Could you check a few things on this model? Use its own coordinates, in mm. A direction names the side the tool comes from. Give positions to 0.01 mm unless a question says otherwise; leave off trailing zeros. Order: outer loops, then holes, each group sorted by start corner. A loop starts at its lowest first (then second) coordinate and runs counter-clockwise, first axis right, second up.
Solid Edge part; units mm, degrees
sketch "Sketch1" plane through (0, 0, 0) normal (1, 0, 0) x (0, 1, 0)
  line L0 (0, 1.95) -> (15, 1.95)
  line L1 (15, 1.95) -> (15, 7.5)
  line L2 (15, 7.5) -> (10.5, 7.5)
  line L3 (10.5, 7.5) -> (10.5, 12.5)
  line L4 (10.5, 12.5) -> (0, 12.5)
  line L5 (0, 12.5) -> (0, 1.95)
  dimension "D1" = 10.5
  dimension "D2" = 15
revolve "RevolvedProtrusion1" add sketch "Sketch1" angle 360 about axis through (0, -60, 0) along (0, 1, 0)
chamfer "Chamfer_1" distance 0.5 angle 60 1 edges at (0, 15, 7.5) measured on face at (-4.85, 15, 5.15)
sketch "Sketch2" plane through (0, 0, 0) normal (0, -1, 0) x (1, 0, 0)
  line L0 (-7.5, 2.5) -> (7.5, 2.5)
  line L1 (7.5, 2.5) -> (10, 35)
  line L2 (10, 95) -> (10, 35)
  line L3 (-10, 95) -> (10, 95)
  line L4 (-10, 35) -> (-10, 95)
  line L5 (-10, 35) -> (-7.5, 2.5)
  dimension "D1" = 10
  dimension "D2" = 7.5
extrude "ExtrudedProtrusion_1" add sketch "Sketch2" against normal blind 9
chamfer "Chamfer_2" distance 0.5 angle 60 1 edges at (0, 0, 1.95) measured on face at (-8.0833, 0, 4.3417)
sketch "Sketch3" plane through (0, 9, 43.7496) normal (0, 1, 0) x (0, 0, -1)
  line L0 (-38.7504, 22.5) -> (-38.7504, -22.5)
  line L1 (-38.7504, -22.5) -> (6.2496, -22.5)
  line L2 (6.2496, -22.5) -> (6.2496, 22.5)
  line L3 (6.2496, 22.5) -> (-38.7504, 22.5)
  dimension "D1" = 38.7504
extrude "ExtrudedProtrusion_2" add sketch "Sketch3" against normal blind 9
sketch "Sketch4" plane through (0, 0, 36.25) normal (0, -1, 0) x (0, 0, 1)
  line L0 (1.25, -22.5) -> (46.25, -22.5)
  line L1 (46.25, -22.5) -> (46.25, 22.5)
  line L2 (46.25, 22.5) -> (1.25, 22.5)
  line L3 (1.25, 22.5) -> (1.25, -22.5)
extrude "ExtrudedCutout_1" cut sketch "Sketch4" against normal blind 3
hole "Hole_1" at (0, 3, 60) direction (0, 1, 0) diameter 8 end up to next
hole "Hole_2" at (15.5, 9, 75.5) direction (0, -1, 0) diameter 3.6 end up to next counterbore diameter 6.5 counterbore depth 4.5
hole "Hole1" at (-15.5, 9, 75.5) direction (0, -1, 0) diameter 3.6 end up to next counterbore diameter 6.5 counterbore depth 4.5
hole "Hole2" at (-15.5, 9, 44.5) direction (0, -1, 0) diameter 3.6 end up to next counterbore diameter 6.5 counterbore depth 4.5
hole "Hole3" at (15.5, 9, 44.5) direction (0, -1, 0) diameter 3.6 end up to next counterbore diameter 6.5 counterbore depth 4.5
sketch "Sketch5" plane through (0, 4.5, 95) normal (0, 0, 1) x (0, 1, 0)
  line L0 (-4.5, 10) -> (0, 10)
  line L1 (0, 10) -> (0, -10)
  line L2 (0, -10) -> (-4.5, -10)
  line L3 (-4.5, -10) -> (-4.5, 10)
extrude "ExtrudedCutout_2" cut sketch "Sketch5" against normal blind 12.5
hole "Hole_6" at (5, 9, 88.75) direction (0, -1, 0) diameter 5 end up to next
hole "Hole4" at (-5, 9, 88.75) direction (0, -1, 0) diameter 5 end up to next
chamfer "Chamfer_3" distance 3 angle 45 4 edges at (22.5, 6, 37.5) (22.5, 6, 82.5) (-22.5, 6, 82.5) (-22.5, 6, 37.5)
chamfer "Chamfer_4" distance 2 angle 45 1 edges at (0, 0, 37.5)
hole "Hole_8" at (0, 3, 60) direction (0, 1, 0) diameter 22 depth 50.8
chamfer "Chamfer_5" distance 0.5 angle 45 1 edges at (0, 3, 71)
properties material "Polyethylene, low density"
Item 1: We'd pull the mould along X, two halves only. Please class faces 1 (the flat face through (10, 7, 89)), 2 (the flat face through (-1.5, 15, 1.5)), 3 (the cylindrical face through (16.717, 3.761, 74.173)): +X half, -X half, draft (parallel to the pull), parting line (faces both ways), or undercut.
Findings:
face 1: +X half
face 2: draft
face 3: undercut
Item 2: Imagine slicing it at B-B on x = 0. Give the number of separate pieces and of enclosed holes in the cut face, then the cut area to 3 significant figures.
Findings:
separate pieces: 3
enclosed holes: 0
area: 688 mm2
Item 3: Please list where these lines run through material, in increasing order: line 1 along Z through (x, y) = (15.5, 6.5); line 2 along X through (y, z) = (3.75, 44.5); line 3 along Z through (x, y) = (15.5, 3.5).
Findings:
line 1: z = 37.5 to 41.25, 47.75 to 72.25, 78.75 to 82.5
line 2: x = -22.5 to -17.3, -13.7 to 13.7, 17.3 to 22.5
line 3: z = 37.5 to 42.7, 46.3 to 73.7, 77.3 to 82.5
Item 4: Imagine slicing it at A-A on z = 75.5. List the corners of the cut face in (x, y) for me, then the cut area to 3 significant figures.
Findings:
outline: (-22.5, 3) - (-17.3, 3) - (-17.3, 4.5) - (-18.75, 4.5) - (-18.75, 9) - (-22.5, 9) - close; (-13.7, 3) - (13.7, 3) - (13.7, 4.5) - (12.25, 4.5) - (12.25, 9) - (-12.25, 9) - (-12.25, 4.5) - (-13.7, 4.5) - close; (17.3, 3) - (22.5, 3) - (22.5, 9) - (18.75, 9) - (18.75, 4.5) - (17.3, 4.5) - close
area: 201 mm2
Item 5: For faces 4 (the flat face through (-8, 10.5, 0)), 5 (the flat face through (10, 3, 70)), 6 (the flat face through (-10, 7, 89)), 7 (the flat face through (-9, 4, 22)), 8 (the cylindrical face through (-14.283, 3.761, 74.173)), which set-ups out of +Z, -Z, +X, -X, +Y, -Y let a thin tool reach every point of the face, with its end or its side?
Findings:
face 4: +Y
face 5: +Z, +X, -X, -Y
face 6: +Z, -X, +Y, -Y
face 7: -X, +Y, -Y
face 8: +Y, -Y
Item 6: For pin 1 (0.8 mm diameter, centred on y = 5, z = 36.5, fed in from +X); pin 2 (10.5 mm diameter, centred on x = 15.5, z = 44.5, fed in from +Y); pin 3 (1.3 mm diameter, centred on y = 7.5, z = 86.5, fed in from -X); pin 4 (3 mm diameter, centred on x = 5, z = 88.75, fed in from -Y), each with a flat end and sliding along its axis, tell me the tip position at first contact or that it passes through.
Findings:
pin 1: stops at x = 10
pin 2: stops at y = 9
pin 3: stops at x = -10
pin 4: passes through
Item 7: Imagine slicing it at C-C on z = 0. List the corners of the cut face in (x, y) for me.
Findings:
outline: (-12.5, 0) - (-2.45, 0) - (-1.95, 0.87) - (-1.95, 15) - (-7, 15) - (-7.5, 14.13) - (-7.5, 10.5) - (-12.5, 10.5) - close; (1.95, 0.87) - (2.45, 0) - (12.5, 0) - (12.5, 10.5) - (7.5, 10.5) - (7.5, 14.13) - (7, 15) - (1.95, 15) - close
